Autodesk Inventor part; units mm, degrees
ref_plane "YZ Plane" through (0, 0, 0) normal (1, 0, 0) x (0, 1, 0)
ref_plane "XZ Plane" through (0, 0, 0) normal (0, 1, 0) x (-1, 0, 0)
ref_plane "XY Plane" through (0, 0, 0) normal (0, 0, 1) x (1, 0, 0)
sketch "Sketch1" plane through (0, 0, 0) normal (1, 0, 0) x (0, 1, 0)
  line L0 (-1.5, 6.858) -> (1.5, 6.858)
  line L1 (1.5, 6.858) -> (1.5, -6.858)
  line L2 (1.5, -6.858) -> (-1.5, -6.858)
  line L3 (-1.5, -6.858) -> (-1.5, 6.858)
  line L4 (-1.5, 6.858) -> (1.5, -6.858) construction
  line L5 (1.5, 6.858) -> (-1.5, -6.858) construction
  line L6 (1.5, 6.858) -> (39.5, 6.858)
  line L7 (39.5, 6.858) -> (39.5, 9.858)
  line L8 (39.5, 9.858) -> (1.5, 9.858)
  line L9 (1.5, 9.858) -> (1.5, 6.858)
  line L10 (1.5, -6.858) -> (39.5, -6.858)
  line L11 (39.5, -6.858) -> (39.5, -9.858)
  line L12 (39.5, -9.858) -> (1.5, -9.858)
  line L13 (1.5, -9.858) -> (1.5, -6.858)
  line L14 (9.5, 6.858) -> (1.5, 6.858)
  line L15 (1.5, 6.858) -> (1.5, -0.142)
  line L16 (1.5, -0.142) -> (9.5, -0.142)
  line L17 (9.5, -0.142) -> (9.5, 6.858)
  line L18 (9.5, -6.858) -> (1.5, -6.858)
  line L19 (1.5, -6.858) -> (1.5, -0.142)
  line L20 (1.5, -0.142) -> (9.5, -0.142)
  line L21 (9.5, -0.142) -> (9.5, -6.858)
  line L22 (9.5, -0.142) -> (1.5, -0.142)
  line L23 (1.5, 6.858) -> (-1.5, 6.858)
  line L24 (-1.5, 6.858) -> (-1.5, 9.858)
  line L25 (-1.5, 9.858) -> (1.5, 9.858)
  line L26 (1.5, 9.858) -> (1.5, 6.858)
  line L27 (1.5, -6.858) -> (-1.5, -6.858)
  line L28 (-1.5, -6.858) -> (-1.5, -9.858)
  line L29 (-1.5, -9.858) -> (1.5, -9.858)
  line L30 (1.5, -9.858) -> (1.5, -6.858)
  point P0 (0, 0)
  dimension "d0" = 3
  dimension "d2" = 13.716
  dimension "d3" = 3
  dimension "d4" = 3
  dimension "d5" = 38
  dimension "d6" = 38
  dimension "d7" = 0
  dimension "d8" = 8
  dimension "d9" = 8
  dimension "d12" = 7
  dimension "d13" = 6.716
extrude "Extrusion1" add sketch "Sketch1" along normal blind 45
sketch "Sketch2" plane through (0, -1.5, 9.858) normal (0, 0, 1) x (1, 0, 0)
  line L0 (5, 7) -> (8.9446, 7)
  arc A0 (5, 7) -> (5, 0) centre (5, 3.5) ccw
  line L1 (8.9446, 0) -> (5, 0)
  arc A1 (13.3822, 14.1239) -> (31.6178, 14.1239) centre (22.5, 3.5) ccw
  line L2 (13.3822, 14.1239) -> (13.3822, 15.7096)
  line L3 (13.6751, 16.4167) -> (15.15, 17.8916)
  arc A2 (13.6751, 16.4167) -> (13.3822, 15.7096) centre (14.3822, 15.7096) ccw
  arc A3 (16.15, 20.3916) -> (15.15, 19.3916) centre (16.15, 19.3916) ccw
  line L4 (15.15, 19.3916) -> (15.15, 17.8916)
  line L5 (28.85, 20.3916) -> (16.15, 20.3916)
  arc A4 (29.85, 19.3916) -> (28.85, 20.3916) centre (28.85, 19.3916) ccw
  line L6 (29.85, 17.8916) -> (29.85, 19.3916)
  line L7 (31.3249, 16.4167) -> (29.85, 17.8916)
  line L8 (31.6178, 15.7096) -> (31.6178, 14.1239)
  arc A5 (31.6178, 15.7096) -> (31.3249, 16.4167) centre (30.6178, 15.7096) ccw
  line L9 (40, 7) -> (36.0554, 7)
  arc A6 (40, 0) -> (40, 7) centre (40, 3.5) ccw
  line L10 (36.0554, 0) -> (40, 0)
  line L11 (40, 7) -> (36.0554, 7)
  arc A7 (40, 0) -> (40, 7) centre (40, 3.5) ccw
  line L12 (36.0554, 0) -> (40, 0)
  line L13 (8.9446, 0) -> (5, 0)
  line L14 (36.0554, 0) -> (40, 0)
  line L15 (0, 41) -> (0, 0)
  line L16 (0, 0) -> (45, 0)
  line L17 (45, 41) -> (45, 0)
  line L18 (0, 41) -> (45, 41)
  line L19 (5, 7) -> (8.9446, 7)
  arc A8 (5, 7) -> (5, 0) centre (5, 3.5) ccw
sketch "Sketch3" plane through (0, -1.5, 9.858) normal (0, 0, 1) x (1, 0, 0)
  line L0 (0, 0) -> (45, 0)
  line L1 (45, 41) -> (45, 0)
  point P0 (0, 41)
  point P1 (0, 1.5)
  point P2 (5, 3.5)
  point P3 (40, 3.5)
  dimension "d16" = 35
  dimension "d18" = 5
  dimension "d19" = 45
  dimension "d20" = 3.5
  dimension "d21" = 3.5
hole "Hole1" at (5, 2, 9.858) at (40, 2, 9.858) direction (0, 0, -1) diameter 4.2 end through all
extrude "Extrusion2" cut sketch "Sketch2" against normal blind 0.82 contours A1 L2 A2 L3 L4 A3 L5 A4 L6 L7 A5 L8 L16 | L16 A1
sketch "Sketch4" plane through (0, -1.5, 9.858) normal (0, 0, 1) x (1, 0, 0)
  arc A0 (36.0554, 0) -> (31.6178, 14.1239) centre (22.5, 3.5) ccw
  line L0 (36.0554, 0) -> (45, 0)
  arc A1 (13.3822, 14.1239) -> (8.9446, 0) centre (22.5, 3.5) ccw
  circle A2 centre (5, 3.5) radius 2.1
  circle A3 centre (40, 3.5) radius 2.1
  arc A4 (5, 7) -> (5, 0) centre (5, 3.5) ccw
  line L1 (5, 7) -> (8.9446, 7)
  line L2 (8.9446, 0) -> (5, 0)
  arc A5 (13.3822, 14.1239) -> (31.6178, 14.1239) centre (22.5, 3.5) ccw
  arc A6 (13.3822, 14.1239) -> (31.6178, 14.1239) centre (22.5, 3.5) ccw
  line L3 (40, 7) -> (36.0554, 7)
  arc A7 (40, 0) -> (40, 7) centre (40, 3.5) ccw
  line L4 (36.0554, 0) -> (40, 0)
  point P0 (0, 1.5)
extrude "Extrusion3" cut sketch "Sketch4" against normal blind 0.82
sketch "Sketch5" plane through (0, -1.5, -9.858) normal (0, 0, -1) x (-1, 0, 0)
  circle A0 centre (-5, 3.5) radius 2.1
  circle A1 centre (-40, 3.5) radius 2.1
  line L0 (-34.959, 3.5) -> (-37.4795, -0.8656)
  line L1 (-37.4795, -0.8656) -> (-42.5205, -0.8656)
  line L2 (-42.5205, -0.8656) -> (-45.041, 3.5)
  line L3 (-45.041, 3.5) -> (-42.5205, 7.8656)
  line L4 (-42.5205, 7.8656) -> (-37.4795, 7.8656)
  line L5 (-37.4795, 7.8656) -> (-34.959, 3.5)
  line L6 (0.041, 3.5) -> (-2.4795, -0.8656)
  line L7 (-2.4795, -0.8656) -> (-7.5205, -0.8656)
  line L8 (-7.5205, -0.8656) -> (-10.041, 3.5)
  line L9 (-10.041, 3.5) -> (-7.5205, 7.8656)
  line L10 (-7.5205, 7.8656) -> (-2.4795, 7.8656)
  line L11 (-2.4795, 7.8656) -> (0.041, 3.5)
  point P0 (0, 1.5)
  point P1 (-40, 3.5)
  point P2 (-5, 3.5)
  dimension "d33" = 8.7312
  dimension "d34" = 8.7312
extrude "Extrusion4" cut sketch "Sketch5" against normal blind 3.175
sketch "Sketch6" plane through (0, 9.5, 6.858) normal (0, 1, 0) x (1, 0, 0)
  line L0 (7.5, 1.82) -> (37.5, 1.82)
  line L1 (37.5, 9.82) -> (7.5, 9.82)
  line L2 (7.5, 1.82) -> (7.5, 9.82)
  line L3 (37.5, 1.82) -> (37.5, 9.82)
  line L4 (7, 10.32) -> (38, 10.32)
  line L5 (38, 10.32) -> (38, 1.32)
  line L6 (38, 1.32) -> (7, 1.32)
  line L7 (7, 1.32) -> (7, 10.32)
  line L8 (8, 10.32) -> (37, 10.32)
  line L9 (37, 10.32) -> (37, 1.32)
  line L10 (37, 1.32) -> (8, 1.32)
  line L11 (8, 1.32) -> (8, 10.32)
  line L12 (0, 0) -> (45, 0)
  line L13 (8, 1.32) -> (37, 1.32)
  line L14 (37, 1.32) -> (37, 0)
  line L15 (37, 0) -> (8, 0)
  line L16 (8, 0) -> (8, 1.32)
  point P0 (0, 6.858)
  dimension "d37" = 0.5
  dimension "d56" = 1
  dimension "d57" = 1
chamfer "Chamfer1" distance 1 angle 45 2 edges at (22.5, 39.5, -6.858) (22.5, 39.5, 6.858)
sketch "Sketch7" plane through (0, 9.5, -6.858) normal (0, 0, 1) x (1, 0, 0)
  line L0 (0, 29) -> (0, 0)
  line L1 (0, 0) -> (45, 0)
  line L2 (45, 29) -> (45, 0)
  circle A0 centre (22.5, 10) radius 4.318
  line L3 (22.5, 10) -> (22.5, 20)
  circle A1 centre (22.5, 20) radius 2.159
  line L4 (20.341, 20) -> (20.341, 6.2605)
  line L5 (24.659, 20) -> (24.659, 6.2605)
  point P0 (0, -9.5)
  dimension "d43" = 8.636
  dimension "d45" = 10
  dimension "d46" = 4.318
  dimension "d47" = 22.5
  dimension "d48" = 45
  dimension "d49" = 10
extrude "Extrusion6" cut sketch "Sketch7" against normal through all
sketch "Sketch8" plane through (0, 9.5, -6.858) normal (0, 0, 1) x (1, 0, 0)
  arc A0 (20.341, 13.7395) -> (24.659, 13.7395) centre (22.5, 10) ccw
  line L0 (20.341, 13.7395) -> (20.341, 20)
  arc A1 (24.659, 20) -> (20.341, 20) centre (22.5, 20) ccw
  line L1 (24.659, 20) -> (24.659, 13.7395)
  line L2 (45, 29) -> (45, 0)
  circle A2 centre (22.5, 20) radius 4.318
  line L3 (18.182, 20) -> (18.182, 10)
  line L4 (26.818, 10) -> (26.818, 20)
  point P0 (0, -9.5)
  dimension "d52" = 4.318
  dimension "d53" = 8.636
extrude "Extrusion7" cut sketch "Sketch8" against normal blind 2 contours L0 A2 L1 A0 | A0 L3 A2 L0 | A2 L1 A1 L0 | A0 L1 A2 L4 picked at (24.9024, 17.6839)
extrude "Extrusion8" cut sketch "Sketch6" against normal through all contours L11 L1 L9 L0 | L0 L9 L6 L11 | L6 L14 L12 L16 | L11 L4 L9 L1
sketch "Sketch9" plane through (0, 0, 0) normal (-1, 0, 0) x (0, 0, 1)
  line L0 (-30, 50) -> (6.858, 50)
  line L1 (6.858, 50) -> (6.858, -18)
  line L2 (6.858, -18) -> (-30, -18)
  line L3 (-30, -18) -> (-30, 50)
  point P0 (0, 0)
extrude "Extrusion9" cut sketch "Sketch9" against normal through all
sketch "Sketch10" plane through (0, -1.5, 9.858) normal (0, 0, 1) x (1, 0, 0)
  line L0 (8, 11) -> (0, 11)
  line L1 (0, 11) -> (0, 0)
  line L2 (0, 0) -> (8, 0)
  line L3 (8, 0) -> (8, 11)
  line L4 (37, 11) -> (45, 11)
  line L5 (45, 11) -> (45, 0)
  line L6 (45, 0) -> (37, 0)
  line L7 (37, 0) -> (37, 11)
  point P0 (0, 1.5)
extrude "Extrusion10" cut sketch "Sketch10" against normal through all
equation "\"d2\" = StretcherDepth"
equation "\"d6\" = d5"
equation "\"d9\" = d8"
equation "\"d47\" = 0.5 * d48"
equation "\"d53\" = 2 * d52"
properties part number "MotorClipV3Front" material "ABS Plastic"
For this review, take the finished solid that the model builds, in its own axes (mm). A direction names the side the tool comes from. Give positions to 0.01 mm unless a question says otherwise; leave off trailing zeros. Write each loop counter-clockwise with the first axis right and the second up, starting at its lowest first coordinate (ties: lowest second). Pieces come first, ordered by that corner, then holes. Notation, with made-up numbers: M -20.75,35 L 12.25,35 A34 ccw 12.25,67 Z; hole C 88,10 d6. An arc over 180 degrees is marked long. Answer as a JSON object with one key per item and string values. Group by question number.
Item 1: Consider section A-A on z = 8.35. Write out the cut boundary in (x, y), plus the area to 3 significant figures.
Item 2: For pin 1 Ø1.5 at (y, z) = (5.5, 9) entering from +X; pin 2 Ø1 at (x, y) = (39.5, 8) entering from -Z; pin 3 Ø0.7 at (x, z) = (21.5, 9.5) entering from -Y; pin 4 Ø16.5 at (x, y) = (24.5, 7.5) entering from +Z, all flat-tipped, find the tip position at first contact; note any pin that passes through.
Item 3: Consider section B-B on x = 22.5. Write out the cut boundary in (y, z).
Item 4: Draft analysis for pull direction X (two halves, no side actions). For faces 1 (the flat face through (14.4, 15.64, 9.45)), 2 (the flat face through (22, 26, 9.858)), 3 (the flat face through (8, 4, 8)), state which applies: +X half, -X half, draft (parallel to the pull), parting line (faces both ways), or undercut.
Item 5: Tool access review of faces 4 (the cylindrical face through (15.451, 18.606, 9.454)), 5 (the flat face through (4, 9.5, 8)), 6 (the flat face through (22.18, 38.99, 7.35)), 7 (the flat face through (41, 9.5, 8)): name each direction out of +Z, -Z, +X, -X, +Y, -Y from which nothing blocks a thin tool from reaching the whole face with its end or side.
Item 6: Consider section D-D on x = 39. Write out the cut boundary in (y, z).
Item 7: Consider section C-C on y = 17. Write out the cut boundary in (x, z), plus the area to 3 significant figures.
Item 8: For probe 1 along Y at (x, z) = (36.5, 9.2); probe 2 along Y at (x, z) = (38, 9.1); probe 3 along Z at (x, y) = (30, 1), list the stretches that pass through material, from the lowest coordinate up. Write a range as [from, to].
Check result:
{
 "1": {"outline": "M 0,9.5 L 8,9.5 L 8,-1.5 L 37,-1.5 L 37,9.5 L 45,9.5 L 45,39.5 L 0,39.5 Z", "area": "1,670 mm^2"},
 "2": {"pin 1": "stops at x = 37", "pin 2": "passes through", "pin 3": "stops at y = 18.89", "pin 4": "stops at z = 9.04"},
 "3": {"outline": "M -1.5,6.86 L 38.5,6.86 L 39.5,7.86 L 39.5,9.86 L 18.89,9.86 L 18.89,9.04 L -1.5,9.04 Z"},
 "4": {"face 1": "undercut", "face 2": "draft", "face 3": "-X half"},
 "5": {"face 4": "+Z, -Y", "face 5": "+Z, -Z, -X, -Y", "face 6": "-Z, +X, -X, +Y", "face 7": "+Z, -Z, +X, -Y"},
 "6": {"outline": "M 9.5,6.86 L 38.5,6.86 L 39.5,7.86 L 39.5,9.86 L 9.5,9.86 Z"},
 "7": {"outline": "M 0,6.86 L 45,6.86 L 45,9.86 L 29.85,9.86 L 29.85,9.04 L 15.15,9.04 L 15.15,9.86 L 0,9.86 Z", "area": "123 mm^2"},
 "8": {"probe 1": "y = [5.5, 39.5]", "probe 2": "y = [9.5, 39.5]", "probe 3": "z = [6.86, 9.04]"}
}
